from build123d import *

# Parameters (mm, degrees)
F1_DEPTH = 25.4
F8_R     = 4.7625
F9_DEPTH = 1828.8


with BuildPart() as f1:
    # F0 (on Front) → F1 (new body)
    with BuildSketch(Plane.XZ):
        Polygon((0, 914.4), (0, 0), (603.25, 0), (603.25, 1822.45), (0, 1822.45), align=None)
    extrude(amount=F1_DEPTH)

    # F5: sweep along a path in F4
    with BuildLine(Plane.XZ.offset(25.4)) as f5_path:
        CenterArc((76.2, 914.4), 21.6276719324, 0, 360)
    # F3 (on offset) → F5 (sweep)
    with BuildSketch(Plane.XY.offset(914.4)):
        with BuildLine():
            Line((57.15, -25.4), (64.6942216848, -53.5554186313))
            ThreePointArc((64.6942216848, -53.5554186313), (51.4984578744, -82.1155571689), (76.2, -101.6))
            Line((76.2, -101.6), (76.2, -25.4))
            Line((76.2, -25.4), (57.15, -25.4))
        make_face()
    sweep(path=f5_path.line)

    # F7: F1 across plane


with BuildPart() as f1_1:
    add(f1.part)
    add(f1.part.mirror(Plane.XZ.offset(12.7)))

    # F8 (on Top) → F9 (join)
    with BuildSketch(Plane.XY):
        with Locations((602.3163199425, -23.3668256551)):
            Circle(F8_R)
    extrude(amount=F9_DEPTH)


solid = f1_1.part
Read the model definition and answer for the solid it produces. Units are mm, in the model's axes. Give positions to 0.01 mm unless a question says otherwise; leave off trailing zeros. Write each loop counter-clockwise with the first axis right and the second up, starting at its lowest first coordinate (ties: lowest second). Pieces come first, ordered by that corner, then holes. Notation, with made-up numbers: (0.5, 36) - (4.5, 36) arc R22 ccw to (4.5, 45) - close; hole circle Ø10 at (31, 20). An arc over 180 degrees is marked (long way). Use CSV: the item, a comma, the result in double quotes. Start each with the question number.
Item 1: Flat-ended cylindrical pins translate along their axes: P1, Ø12, axis at x = 331, z = 1509.5, coming from the +Y side; P2, Ø6, axis at x = 435.5, z = 962.5, coming from the -Y side; P3, Ø6, axis at y = -3, z = 952.5, coming from the +X side. Find the tip coordinate at first contact, or state that the pin passes through.
Item 2: The part is cut by section B-B, the plane x = 557. Give the vertices of the cut face in (y, z).
Item 3: Consider line 1 (Z direction, x = 331.5, y = -11); line 2 (Y direction, x = 236, z = 535.5); line 3 (X direction, y = -23.5, z = 126). Determine where each line is inside the solid, lowest interval first.
Taken from the geometry:
1,P1,"y = 0"
1,P2,"y = -25.4"
1,P3,"x = 603.25"
2,outline,"(-25.4, 0) - (0, 0) - (0, 1822.45) - (-25.4, 1822.45) - close"
3,line 1,"0 to 1822.45"
3,line 2,"-25.4 to 0"
3,line 3,"0 to 607.08"
